from build123d import *

# Parameters (mm, degrees)
SKETCH_1_R      = 3
EXTRUDE_1_DEPTH = 20


with BuildPart() as part:
    # 草图1 → 凸台-拉伸1 (new body)
    with BuildSketch(Plane(origin=(0, 0, 0), x_dir=(1, 0, 0), z_dir=(0, 1, 0))):
        Polygon((0, 0), (264, 0), (264, 60), (224, 60), (224, 84), (204, 84), (204, 60), (174, 60), (174, 14.075760101), (90, 14.075760101), (90, 60), (60, 60), (60, 84), (40, 84), (40, 60), (0, 60), align=None)
        with Locations((13, 36)):
            Circle(SKETCH_1_R, mode=Mode.SUBTRACT)
        with Locations((79, 22)):
            Circle(SKETCH_1_R, mode=Mode.SUBTRACT)
        with Locations((195, 22)):
            Circle(SKETCH_1_R, mode=Mode.SUBTRACT)
        with Locations((250, 36)):
            Circle(SKETCH_1_R, mode=Mode.SUBTRACT)
        with BuildLine():
            Line((37.266898407, 43.924239899), (63.266898407, 29.924239899))
            ThreePointArc((63.266898407, 29.924239899), (66.924239899, 17.733101593), (54.733101593, 14.075760101))
            Line((54.733101593, 14.075760101), (28.733101593, 28.075760101))
            ThreePointArc((28.733101593, 28.075760101), (25.075760101, 40.266898407), (37.266898407, 43.924239899))
        make_face(mode=Mode.SUBTRACT)
        with BuildLine():
            Line((208.859135747, 28.579497414), (223.859135747, 42.579497414))
            ThreePointArc((223.859135747, 42.579497414), (236.579497414, 42.140864253), (236.140864253, 29.420502586))
            Line((236.140864253, 29.420502586), (221.140864253, 15.420502586))
            ThreePointArc((221.140864253, 15.420502586), (208.420502586, 15.859135747), (208.859135747, 28.579497414))
        make_face(mode=Mode.SUBTRACT)
    extrude(amount=EXTRUDE_1_DEPTH)


solid = part.part
Design review of the part built by this model. Coordinates are the model's own, in mm. A direction names the side the tool comes from. Coordinates: 2 decimals unless noted, no trailing zeros. Loops run counter-clockwise (first coordinate to the right, second up) from the corner with the lowest first, then second, coordinate; pieces in that order, holes last. Notation, with made-up numbers: M 0.25,-14 L 21.25,-14 A15 ccw 21.25,-1 Z; hole C 20,23 d3. An arc over 180 degrees is marked long. Use one line per item in the form item = value.
(1) Draft analysis for pull direction Z (two halves, no side actions). For faces 1 (the face through (90, 10, -37)), 2 (the face through (189, 10, -60)), 3 (the face through (197.86, 9.86, -22.9)), state which applies: pulls with the +Z half, pulls with the -Z half, needs draft (parallel to the pull), parting line crosses it, or undercut.
Return value:
face_1 = needs draft
face_2 = pulls with the -Z half
face_3 = undercut
(2) Consider section A-A (x = 79). Write out the cut boundary in (y, z), and give its area (3 significant figures).
Return value:
outline = M 0,-60 L 20,-60 L 20,-25 L 0,-25 Z; M 0,-19 L 20,-19 L 20,0 L 0,0 Z
area = 1,080 mm2
(3) Consider section B-B (z = -72). Write out the cut boundary in (x, y).
Return value:
outline = M 40,0 L 60,0 L 60,20 L 40,20 Z; M 204,0 L 224,0 L 224,20 L 204,20 Z
(4) Consider section D-D (z = -22). Write out the cut boundary in (x, y).
Return value:
outline = M 0,0 L 40.02,0 L 40.02,20 L 0,20 Z; M 68,0 L 76,0 L 76,20 L 68,20 Z; M 82,0 L 90,0 L 90,20 L 82,20 Z; M 174,0 L 192,0 L 192,20 L 174,20 Z; M 198,0 L 206,0 L 206,20 L 198,20 Z; M 228.19,0 L 264,0 L 264,20 L 228.19,20 Z
(5) For faces 4 (the face through (41.915, 9.86, -20.978)), 5 (the face through (75, 10, -60)), 6 (the face through (20, 10, -60)), list the 3-axis set-ups (+Z, -Z, +X, -X, +Y, -Y) from which the entire face can be reached by the end or side of a thin tool; tool diameter is ignored.
Return value:
face_4 = +Y, -Y
face_5 = -Z, +Y, -Y
face_6 = -Z, -X, +Y, -Y
(6) Consider section C-C (y = 8). Write out the cut boundary in (x, z).
Return value:
outline = M 0,-60 L 40,-60 L 40,-84 L 60,-84 L 60,-60 L 90,-60 L 90,-14.08 L 174,-14.08 L 174,-60 L 204,-60 L 204,-84 L 224,-84 L 224,-60 L 264,-60 L 264,0 L 0,0 Z; hole C 13,-36 d6; hole M 28.73,-28.08 A9 ccw 37.27,-43.92 L 63.27,-29.92 A9 ccw 54.73,-14.08 Z; hole C 79,-22 d6; hole C 195,-22 d6; hole M 208.86,-28.58 L 223.86,-42.58 A9 ccw 236.14,-29.42 L 221.14,-15.42 A9 ccw Z; hole C 250,-36 d6
(7) Clearance check with flat-ended pins moving along their axes: P1, Ø10, axis at x = 241.5, y = 12.5, coming from the -Z side; P2, Ø6, axis at y = 11.5, z = -74.5, coming from the +X side; P3, Ø10, axis at x = 114.5, y = 5, coming from the -Z side. State where each tip first meets the part, or that it passes through.
Return value:
P1 = -60
P2 = 224
P3 = -14.08
(8) For line 1 along Z through (x, y) = (13, 12.5); line 2 along X through (y, z) = (12.25, -36); line 3 along Z through (x, y) = (79, 6), list the stretches that pass through material, from the lowest coordinate up. Write a range as from..to.
Return value:
line_1 = -60..-39, -33..0
line_2 = 0..10, 16..24, 51.98..90, 174..216.81, 239..247, 253..264
line_3 = -60..-25, -19..0
